Design review of the part built by this model. Coordinates are the model's own, in mm. Coordinates: 2 decimals unless noted, no trailing zeros. Loops run counter-clockwise (first coordinate to the right, second up) from the corner with the lowest first, then second, coordinate; pieces in that order, holes last. Notation, with made-up numbers: (51, 79) -> (94, 79) arc R28 cw to (94, 113) -> close; hole circle Ø7 at (-15, -39.5). An arc over 180 degrees is marked (long way). Use a Markdown table: item, result. Add a question column.
Q1. Take a section at D-D on x = 12. Write out the cut boundary in (y, z), plus the area to 3 significant figures.
Q2. Clearance check with flat-ended pins moving along their axes: pin 1 Ø2 at (x, y) = (-24.5, 3) entering from +Z; pin 2 Ø2 at (y, z) = (2.5, 35) entering from -X; pin 3 Ø1.7 at (x, y) = (25, 5) entering from +Z; pin 4 Ø1.5 at (y, z) = (3.5, 33.5) entering from +X. State where each tip first meets the part, or that it passes through.
Q3. For probe 1 along Y at (x, z) = (15, 35.15); probe 2 along Y at (x, z) = (25, 32); probe 3 along X at (y, z) = (6.25, 31.55), list the stretches that pass through material, from the lowest coordinate up.
Q4. Take a section at A-A on z = 35.15. Count the separate pieces of the cut face and the enclosed holes in it, plus the area to 3 significant figures.
Q5. Take a section at B-B on x = -25. Write out the cut boundary in (y, z), plus the area to 3 significant figures.
Q6. Take a section at C-C on y = 7. Write out the cut boundary in (x, z), plus the area to 3 significant figures.
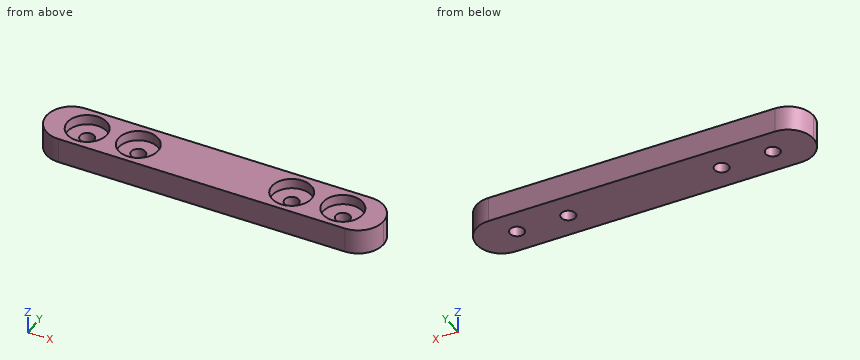
from build123d import *

# Parameters (mm, degrees)
SKETCH1_W               = 66
SKETCH1_H               = 72
BOSS_EXTRUDE1_DEPTH     = 10
SKETCH2_R               = 1.4
CUT_EXTRUDE1_DEPTH      = 10
CUT_EXTRUDE2_DEPTH      = 50.849774322
CUT_EXTRUDE2_DEPTH_BACK = 50.849774322
SKETCH3_W               = 30
SKETCH3_H               = 5
SKETCH5_R               = 7.5
BOSS_EXTRUDE2_DEPTH     = 1.5
SKETCH6_W               = 67
SKETCH6_H               = 25
CUT_EXTRUDE4_DEPTH      = 77.054256949
FILLET1_R               = 5
SKETCH7_R               = 3.9
SKETCH7_R_2             = 1.4
CUT_EXTRUDE5_DEPTH      = 2


with BuildPart() as part:
    # Sketch1 → Boss-Extrude1 (new body)
    with BuildSketch(Plane(origin=(0, 0, 0), x_dir=(1, 0, 0), z_dir=(0, 1, 0))):
        Rectangle(SKETCH1_W, SKETCH1_H)
    extrude(amount=BOSS_EXTRUDE1_DEPTH)

    # Sketch2 → Cut-Extrude1 (cut)
    with BuildSketch(Plane.XY.offset(36)):
        with Locations((-15, 5)):
            Circle(SKETCH2_R)
        with Locations((15, 5)):
            Circle(SKETCH2_R)
        with Locations((-25, 5)):
            Circle(SKETCH2_R)
        with Locations((25, 5)):
            Circle(SKETCH2_R)
    cut_extrude1 = extrude(amount=-CUT_EXTRUDE1_DEPTH, mode=Mode.SUBTRACT)

    # Mirror1: Cut-Extrude1 across plane
    add(cut_extrude1.mirror(Plane.XY), mode=Mode.SUBTRACT)

    # Sketch3 → Cut-Extrude2 (cut, two sides: drawn at the far end of the back side and taken through both)
    with BuildSketch(Plane(origin=(0, 10, 0), x_dir=(1, 0, 0), z_dir=(0, 1, 0)).offset(-CUT_EXTRUDE2_DEPTH_BACK)):
        with Locations((0, -19)):
            Rectangle(SKETCH3_W, SKETCH3_H)
        with Locations((0, 19)):
            Rectangle(SKETCH3_W, SKETCH3_H)
    extrude(amount=CUT_EXTRUDE2_DEPTH + CUT_EXTRUDE2_DEPTH_BACK, mode=Mode.SUBTRACT)

    # Sketch5 → Boss-Extrude2 (add)
    with BuildSketch(Plane(origin=(0, 10, 0), x_dir=(1, 0, 0), z_dir=(0, 1, 0))):
        with Locations(Location((0, 0, 0), (0, 0, 270))):
            Circle(SKETCH5_R)
    extrude(amount=BOSS_EXTRUDE2_DEPTH)

    # Sketch6 → Cut-Extrude4 (cut, through all)
    with BuildSketch(Plane(origin=(33, 0, 0), x_dir=(0, 0, -1), z_dir=(1, 0, 0))):
        with Locations((2.5, 12.5)):
            Rectangle(SKETCH6_W, SKETCH6_H)
    extrude(amount=-CUT_EXTRUDE4_DEPTH, mode=Mode.SUBTRACT)

    # Fillet1
    fillet1_edges = [part.edges().sort_by_distance(p)[0] for p in [
        (33, 0, 33.5),
        (33, 10, 33.5),
        (-33, 0, 33.5),
        (-33, 10, 33.5),
    ]]
    fillet(fillet1_edges, radius=FILLET1_R - 0.0001)  # a hair under: the kernel refuses the full size

    # Sketch7 → Cut-Extrude5 (cut)
    # profile 1 of 4: a face of its own
    with BuildSketch(Plane.XY.offset(36)):
        with Locations((-25, 5)):
            Circle(SKETCH7_R)
        with Locations((-25, 5)):
            Circle(SKETCH7_R_2, mode=Mode.SUBTRACT)
    # profile 2 of 4: a face of its own
    with BuildSketch(Plane.XY.offset(36)):
        with Locations((-15, 5)):
            Circle(SKETCH7_R)
        with Locations((-15, 5)):
            Circle(SKETCH7_R_2, mode=Mode.SUBTRACT)
    # profile 3 of 4: a face of its own
    with BuildSketch(Plane.XY.offset(36)):
        with Locations((15, 5)):
            Circle(SKETCH7_R)
        with Locations((15, 5)):
            Circle(SKETCH7_R_2, mode=Mode.SUBTRACT)
    # profile 4 of 4: a face of its own
    with BuildSketch(Plane.XY.offset(36)):
        with Locations((25, 5)):
            Circle(SKETCH7_R)
        with Locations((25, 5)):
            Circle(SKETCH7_R_2, mode=Mode.SUBTRACT)
    extrude(amount=-CUT_EXTRUDE5_DEPTH, mode=Mode.SUBTRACT)


solid = part.part
Answer list:
| question | item | result |
|---|---|---|
| 1 | outline | (0, 31) -> (10, 31) -> (10, 36) -> (7.49, 36) -> (7.49, 34) -> (2.51, 34) -> (2.51, 36) -> (0, 36) -> close |
| 1 | area | 40.0 mm² |
| 2 | pin 1 | z = 34 |
| 2 | pin 2 | x = -32.77 |
| 2 | pin 3 | through |
| 2 | pin 4 | x = 32.94 |
| 3 | probe 1 | 0 to 1.1, 8.9 to 10 |
| 3 | probe 2 | 0 to 3.6, 6.4 to 10 |
| 3 | probe 3 | -32.84 to -25.63, -24.37 to -15.63, -14.37 to 14.37, 15.63 to 24.37, 25.63 to 32.84 |
| 4 | separate pieces | 1 |
| 4 | enclosed holes | 4 |
| 4 | area | 447 mm² |
| 5 | outline | (0, 31) -> (3.6, 31) -> (3.6, 34) -> (1.1, 34) -> (1.1, 36) -> (0, 36) -> close; (6.4, 31) -> (10, 31) -> (10, 36) -> (8.9, 36) -> (8.9, 34) -> (6.4, 34) -> close |
| 5 | area | 26.0 mm² |
| 6 | outline | (-32.58, 31) -> (32.58, 31) -> (32.58, 36) -> (28.35, 36) -> (28.35, 34) -> (21.65, 34) -> (21.65, 36) -> (18.35, 36) -> (18.35, 34) -> (11.65, 34) -> (11.65, 36) -> (-11.65, 36) -> (-11.65, 34) -> (-18.35, 34) -> (-18.35, 36) -> (-21.65, 36) -> (-21.65, 34) -> (-28.35, 34) -> (-28.35, 36) -> (-32.58, 36) -> close |
| 6 | area | 272 mm² |
